```python
from build123d import *

# Parameters (mm, degrees)
SKETCH1_R           = 6
SKETCH1_R_2         = 1.25
SKETCH1_R_3         = 1.5
BOSS_EXTRUDE1_DEPTH = 5


with BuildPart() as part:
    # Sketch1 → Boss-Extrude1 (new body)
    with BuildSketch(Plane.XY):
        Polygon((0, -2.857142857), (40, -2.857142857), (40, 37.142857143), (40, 43.840888812), (0, 43.840888812), (0, 37.142857143), align=None)
        with Locations((20, 7.142857143)):
            Circle(SKETCH1_R, mode=Mode.SUBTRACT)
        with Locations((4.491483608, 14.123968753)):
            Circle(SKETCH1_R_2, mode=Mode.SUBTRACT)
        with Locations((12.257831183, 0.710026553)):
            Circle(SKETCH1_R_2, mode=Mode.SUBTRACT)
        with Locations((27.757819681, 0.728909749)):
            Circle(SKETCH1_R_2, mode=Mode.SUBTRACT)
        with Locations((35.491460603, 14.161735143)):
            Circle(SKETCH1_R_2, mode=Mode.SUBTRACT)
        with Locations((10, 38.807411058)):
            Circle(SKETCH1_R_3, mode=Mode.SUBTRACT)
        with Locations(Location((30, 38.807411058, 0), (0, 0, 180))):
            Circle(SKETCH1_R_3, mode=Mode.SUBTRACT)
    extrude(amount=BOSS_EXTRUDE1_DEPTH)


solid = part.part
```
Part model, mm, in its own coordinate system. Round coordinates to 2 decimals unless told otherwise and drop trailing zeros. Loops run counter-clockwise (first coordinate to the right, second up) from the corner with the lowest first, then second, coordinate; pieces in that order, holes last.
Item 1: Cut at C-C, the plane z = 4.2. Give the cut face in (x, y), then the cut area to 3 significant figures.
Item 2: Cut at B-B, the plane y = 3.5. Give the cut face in (x, z), then the cut area to 3 significant figures.
Item 3: Drop a flat-ended pin along its axis: P1, Ø11, axis at x = 20, y = 7.14, coming from the +Z side. Give the stop position or say it passes through.
Item 4: Cut at A-A, the plane x = 20. Give the cut face in (y, z), then the cut area to 3 significant figures.
Item 5: Mould opens along Y. For faces 1 (the face through (20, 21, 0)), 2 (the face through (22.77, 1.82, 2.46)), 3 (the face through (20, -2.857, 2)) say: +Y half, -Y half, draft (parallel to the pull), parting line (faces both ways), or undercut.
Item 6: Drill centre lines: line 1 (X direction, y = 0.5, z = 1.5); line 2 (Y direction, x = 35.5, z = 4.3); line 3 (X direction, y = 40, z = 2.2). Where is each one in solid material? Low to high.
A:
1. outline: (0, -2.86) - (40, -2.86) - (40, 43.84) - (0, 43.84) - close; hole circle Ø2.5 at (4.49, 14.12); hole circle Ø3 at (10, 38.81); hole circle Ø2.5 at (12.26, 0.71); hole circle Ø12 at (20, 7.14); hole circle Ø2.5 at (27.76, 0.73); hole circle Ø3 at (30, 38.81); hole circle Ø2.5 at (35.49, 14.16)
1. area: 1,720 mm2
2. outline: (0, 0) - (15.23, 0) - (15.23, 5) - (0, 5) - close; (24.77, 0) - (40, 0) - (40, 5) - (24.77, 5) - close
2. area: 152 mm2
3. P1: passes through
4. outline: (-2.86, 0) - (1.14, 0) - (1.14, 5) - (-2.86, 5) - close; (13.14, 0) - (43.84, 0) - (43.84, 5) - (13.14, 5) - close
4. area: 173 mm2
5. face 1: draft
5. face 2: undercut
5. face 3: -Y half
6. line 1: x = 0 to 11.03, 13.49 to 26.53, 28.99 to 40
6. line 2: y = -2.86 to 12.91, 15.41 to 43.84
6. line 3: x = 0 to 9.09, 10.91 to 29.09, 30.91 to 40
